For this review, take the finished solid that the model builds, in its own axes (mm). Face numbers are marked on the shaded views. A direction names the side the tool comes from. Round coordinates to 2 decimals unless told otherwise and drop trailing zeros. Order: outer loops, then holes, each group sorted by start corner. A loop starts at its lowest first (then second) coordinate and runs counter-clockwise, first axis right, second up. Notation, with made-up numbers: (-35, -34.5) - (15, -34.5) arc R21 ccw to (15, -26.5) - close; hole circle Ø8 at (32.25, -36). An arc over 180 degrees is marked (long way). One line per item, written item: value.
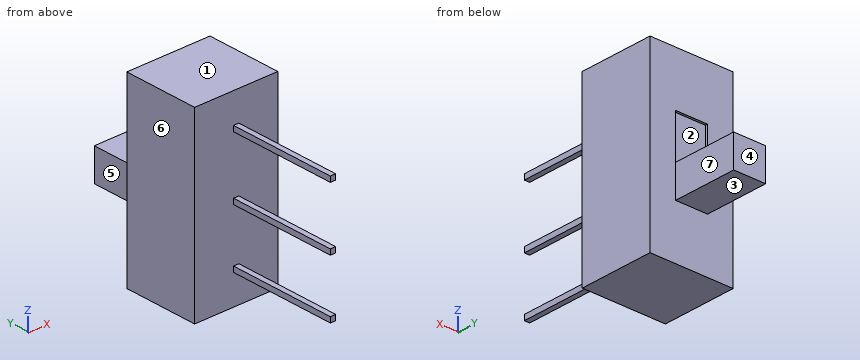
```python
from build123d import *

# Parameters (mm, degrees)
SKETCH1_W           = 3.9
SKETCH1_H           = 8.55
BOSS_EXTRUDE1_DEPTH = 3.5
SKETCH2_W           = 1.5
SKETCH2_H           = 3
BOSS_EXTRUDE2_DEPTH = 1.5
SKETCH3_W           = 2.05
SKETCH3_H           = 0.11
CUT_EXTRUDE1_DEPTH  = 1.5
SKETCH4_W           = 0.25
SKETCH4_H           = 0.25
BOSS_EXTRUDE3_DEPTH = 5
SKETCH5_W           = 0.25
SKETCH5_H           = 0.25
BOSS_EXTRUDE4_DEPTH = 5
SKETCH6_W           = 0.25
SKETCH6_H           = 0.25
BOSS_EXTRUDE5_DEPTH = 5


with BuildPart() as part:
    # Sketch1 → Boss-Extrude1 (new body)
    with BuildSketch(Plane(origin=(0, 3.5, 0), x_dir=(1, 0, 0), z_dir=(0, 1, 0))):
        with Locations((1.95, 4.275)):
            Rectangle(SKETCH1_W, SKETCH1_H)
    extrude(amount=-BOSS_EXTRUDE1_DEPTH)

    # Sketch2 → Boss-Extrude2 (add)
    with BuildSketch(Plane(origin=(2.7, 0, 0), x_dir=(0, 0, -1), z_dir=(1, 0, 0))):
        with Locations((5.3, 5)):
            Rectangle(SKETCH2_W, SKETCH2_H)
    extrude(amount=-BOSS_EXTRUDE2_DEPTH)

    # Sketch3 → Cut-Extrude1 (cut)
    with BuildSketch(Plane(origin=(2.7, 0, 0), x_dir=(0, 0, -1), z_dir=(1, 0, 0))):
        with Locations((3.525, 3.445)):
            Rectangle(SKETCH3_W, SKETCH3_H)
    extrude(amount=-CUT_EXTRUDE1_DEPTH, mode=Mode.SUBTRACT)

    # Sketch4 → Boss-Extrude3 (add)
    with BuildSketch(Plane.XZ):
        with Locations((1.95, -7.05)):
            Rectangle(SKETCH4_W, SKETCH4_H)
    extrude(amount=BOSS_EXTRUDE3_DEPTH)

    # Sketch5 → Boss-Extrude4 (add)
    with BuildSketch(Plane.XZ):
        with Locations((1.95, -1.5)):
            Rectangle(SKETCH5_W, SKETCH5_H)
    extrude(amount=BOSS_EXTRUDE4_DEPTH)

    # Sketch6 → Boss-Extrude5 (add)
    with BuildSketch(Plane.XZ):
        with Locations((1.95, -4.375)):
            Rectangle(SKETCH6_W, SKETCH6_H)
    extrude(amount=BOSS_EXTRUDE5_DEPTH)


solid = part.part
```
Item 1: Take a section at D-D (z = -3.5). Write out the cut boundary in (x, y).
Returned:
outline: (0, 0) - (3.9, 0) - (3.9, 3.5) - (2.7, 3.5) - (2.7, 3.39) - (1.2, 3.39) - (1.2, 3.5) - (0, 3.5) - close
Item 2: The part is to be moulded in two halves that separate along Z. For the marked faces 1, 2, 3 and 4, say which applies: +Z half, -Z half, draft (parallel to the pull), parting line (faces both ways), or undercut.
Returned:
face 1: +Z half
face 2: undercut
face 3: -Z half
face 4: draft
Item 3: Take a section at C-C (x = 2.2). Write out the cut boundary in (y, z), plus the area to 3 significant figures.
Returned:
outline: (0, -8.55) - (3.5, -8.55) - (3.5, -6.05) - (6.5, -6.05) - (6.5, -4.55) - (3.39, -4.55) - (3.39, -2.5) - (3.5, -2.5) - (3.5, 0) - (0, 0) - close
area: 34.2 mm^2
Item 4: Take a section at A-A (y = -1.5). Write out the cut boundary in (x, z) (3 decimals).
Returned:
outline: (1.825, -7.175) - (2.075, -7.175) - (2.075, -6.925) - (1.825, -6.925) - close; (1.825, -4.5) - (2.075, -4.5) - (2.075, -4.25) - (1.825, -4.25) - close; (1.825, -1.625) - (2.075, -1.625) - (2.075, -1.375) - (1.825, -1.375) - close
Item 5: Machinability: for the marked faces 5, 6 and 7, which of the approach directions +Z, -Z, +X, -X, +Y, -Y give a long, thin tool a straight path to every point of the face, cutting with its end or side? Answer none if there is none.
Returned:
face 5: +Z, -Z, -X, +Y
face 6: +Z, -Z, -X, +Y, -Y
face 7: +Z, -Z, +X, +Y
Item 6: Wall thickness on line 1 (Y direction, x = 0.7, z = -5.25); line 2 (X direction, y = -1.25, z = -7) (3 decimals); line 3 (Y direction, x = 2.05, z = -3.5): over which ranges is each line inside the solid? List them lowest first.
Returned:
line 1: 0 to 3.5
line 2: 1.825 to 2.075
line 3: 0 to 3.39
Item 7: For P1, Ø1, axis at x = 3, z = -7, coming from the -Y side; P2, Ø1.6, axis at x = 2, y = 5, coming from the +Z side; P3, Ø2, axis at y = 5, z = -6.5, coming from the +X side, all flat-tipped, find the tip position at first contact; note any pin that passes through.
Returned:
P1: y = 0
P2: z = -4.55
P3: x = 2.7
Item 8: Take a section at B-B (z = -5). Write out the cut boundary in (x, y), plus the area to 4 significant figures.
Returned:
outline: (0, 0) - (3.9, 0) - (3.9, 3.5) - (2.7, 3.5) - (2.7, 6.5) - (1.2, 6.5) - (1.2, 3.5) - (0, 3.5) - close
area: 18.15 mm^2
